```python
from build123d import *

# Parameters (mm, degrees)
SKETCH1_R               = 50.8
SKETCH1_R_2             = 49.6697
BOSS_EXTRUDE1_DEPTH     = 1320.8
CUT_EXTRUDE1_REACH      = 1327.676
CUT_EXTRUDE1_END_RADIUS = 49.6697
CIRPATTERN1_COUNT       = 3


with BuildPart() as part:
    # Sketch1 → Boss-Extrude1 (new body)
    with BuildSketch(Plane.XY):
        Circle(SKETCH1_R)
        Circle(SKETCH1_R_2, mode=Mode.SUBTRACT)
    extrude(amount=BOSS_EXTRUDE1_DEPTH)

    # Cut-Extrude1: up to this cylinder (the profile starts outside it)
    cut_extrude1_end = Plane(origin=(0, 0, 160.782), z_dir=(0, 0, -1)) * Cylinder(CUT_EXTRUDE1_END_RADIUS, 2755.6914, mode=Mode.PRIVATE)
    # Sketch2 → Cut-Extrude1 (cut, up to the surface)
    with BuildSketch(Plane(origin=(50.8, 0, 0), x_dir=(0, 0, -1), z_dir=(1, 0, 0)), mode=Mode.PRIVATE) as cut_extrude1_sk1:
        with BuildLine():
            Line((-8.382, -2.38125), (-313.182, -2.38125))
            ThreePointArc((-313.182, -2.38125), (-315.56325, 0), (-313.182, 2.38125))
            Line((-313.182, 2.38125), (-8.382, 2.38125))
            ThreePointArc((-8.382, 2.38125), (-6.00075, 0), (-8.382, -2.38125))
        make_face()
    cut_extrude1_tool1 = extrude(cut_extrude1_sk1.sketch, amount=-CUT_EXTRUDE1_REACH, mode=Mode.PRIVATE) - cut_extrude1_end
    cut_extrude1 = cut_extrude1_tool1.solids().sort_by_distance((50.8, 0, 160.782))[0]
    add(cut_extrude1, mode=Mode.SUBTRACT)

    # CirPattern1: Cut-Extrude1 ×3 about axis
    cirpattern1_axis = Axis((0, 0, 0), (0, 0, 1))
    for i in range(1, CIRPATTERN1_COUNT):
        add(cut_extrude1.rotate(cirpattern1_axis, i * 360 / CIRPATTERN1_COUNT), mode=Mode.SUBTRACT)


solid = part.part
```
Design review of the part built by this model. Coordinates are the model's own, in mm. Coordinates: 2 decimals unless noted, no trailing zeros. Write each loop counter-clockwise with the first axis right and the second up, starting at its lowest first coordinate (ties: lowest second). Pieces come first, ordered by that corner, then holes. Notation, with made-up numbers: M -37.75,61 L 7.25,61 A15 ccw 7.25,81 Z; hole C -30,-7 d9. An arc over 180 degrees is marked long. Answer as a JSON object with one key per item and string values.
Item 1: Wall thickness on probe 1 along Y at (x, z) = (2.5, 996); probe 2 along Y at (x, z) = (-4, 59); probe 3 along X at (y, z) = (10, 60.5): over which ranges is each line inside the solid? List them lowest first.
Outcome:
{"probe 1": "-50.74 to -49.61, 49.61 to 50.74", "probe 2": "-50.64 to -49.51, 49.51 to 50.64", "probe 3": "-49.81 to -48.65, 48.65 to 49.81"}
Item 2: Draft analysis for pull direction X (two halves, no side actions). For faces 1 (the cylindrical face through (22.92, -44.066, 651.154)), 2 (the cylindrical face through (-11.012, -49.592, 651.154)), 3 (the flat face through (11, -49, 0)), state which applies: pulls with the +X half, pulls with the -X half, needs draft (parallel to the pull), parting line crosses it, or undercut.
Outcome:
{"face 1": "undercut", "face 2": "parting line crosses it", "face 3": "needs draft"}
Item 3: Add section C-C, the plane z = 447. Give the boundary of the cut face in (x, y), and give its area (3 significant figures).
Outcome:
{"outline": "C 0,0 d101.6; hole C 0,0 d99.34", "area": "357 mm²"}
Item 4: Add section A-A, the plane x = 0. Give the boundary of the cut face in (y, z), and give its area (3 significant figures).
Outcome:
{"outline": "M -50.8,0 L -49.67,0 L -49.67,1320.8 L -50.8,1320.8 Z; M 49.67,0 L 50.8,0 L 50.8,1320.8 L 49.67,1320.8 Z", "area": "2,990 mm²"}
Item 5: Insertion check: pin 1 Ø1 at (x, z) = (23.5, 256.5) entering from -Y; pin 2 Ø1 at (y, z) = (19, 1165) entering from +X; pin 3 Ø10 at (x, z) = (15, 1105.5) entering from +Y. Each pin has a flat end and moves straight along its axis. Give the tip position at first contact, or say it passes through.
Outcome:
{"pin 1": "y = -45.3", "pin 2": "x = 47.31", "pin 3": "y = 49.81"}
Item 6: Add section B-B, the plane y = 16. Give the boundary of the cut face in (x, z), and give its area (3 significant figures).
Outcome:
{"outline": "M -48.21,0 L -47.02,0 L -47.02,1320.8 L -48.21,1320.8 Z; M 47.02,0 L 48.21,0 L 48.21,1320.8 L 47.02,1320.8 Z", "area": "3,150 mm²"}
